from build123d import *

# Parameters (mm, degrees)
F1_DEPTH = 10
F3_DEPTH = 9
F4_R     = 2.5
F5_DEPTH = 9


with BuildPart() as f1:
    # F0 (on Right) → F1 (new body)
    with BuildSketch(Plane.YZ):
        Polygon((2.31229, 22.044512), (-24.890254, 22.044512), (-24.890254, 13.044512), (-0.099253, 13.044512), (23.129309, -0.366504), (27.629309, 7.427725), align=None)
    extrude(amount=F1_DEPTH)

    # F2 (on face) → F3 (join)
    with BuildSketch(Plane(origin=(0, 0, 13.044512), x_dir=(1, 0, 0), z_dir=(0, 0, -1))):
        with BuildLine():
            Line((0, 24.890254), (10, 24.890254))
            ThreePointArc((10, 24.890254), (5, 29.890254), (0, 24.890254))
        make_face()
    extrude(amount=-F3_DEPTH)

    # F4 (on face) → F5 (cut)
    with BuildSketch(Plane(origin=(0, 0, 13.044512), x_dir=(1, 0, 0), z_dir=(0, 0, -1))):
        with Locations((5, 24.890254)):
            Circle(F4_R)
    extrude(amount=-F5_DEPTH, mode=Mode.SUBTRACT)


solid = f1.part
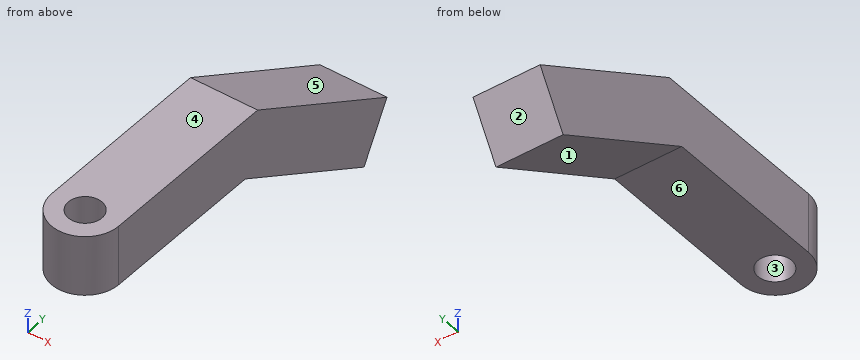
Part model, mm, in its own coordinate system. Face numbers are marked on the shaded views. A direction names the side the tool comes from. Give positions to 0.01 mm unless a question says otherwise; leave off trailing zeros. Order: outer loops, then holes, each group sorted by start corner. A loop starts at its lowest first (then second) coordinate and runs counter-clockwise, first axis right, second up. Notation, with made-up numbers: (-20.75, 50) - (-4.75, 50) arc R16 ccw to (-4.75, 67) - close; hole circle Ø6 at (7, 14). An arc over 180 degrees is marked (long way). Use a Markdown table: item, result.
1) Saw through at D-D on x = 1. List the corners of the cut face in (y, z), plus the area to 3 significant figures.
Checked values:
| item | result |
|---|---|
| outline | (-27.89, 13.04) - (-0.1, 13.04) - (23.13, -0.37) - (27.63, 7.43) - (2.31, 22.04) - (-27.89, 22.04) - close |
| area | 513 mm² |
2) 3-axis set-ups, long thin cutter, end or side, ignore diameter. For the marked faces 5 and 6: which of +Z, -Z, +X, -X, +Y, -Y reach the whole face in a straight line?
Checked values:
| item | result |
|---|---|
| face 5 | +Z, +X, -X, +Y |
| face 6 | -Z, +X, -X, -Y |
3) Saw through at A-A on x = 5. List the corners of the cut face in (y, z).
Checked values:
| item | result |
|---|---|
| outline | (-29.89, 13.04) - (-27.39, 13.04) - (-27.39, 22.04) - (-29.89, 22.04) - close; (-22.39, 13.04) - (-0.1, 13.04) - (23.13, -0.37) - (27.63, 7.43) - (2.31, 22.04) - (-22.39, 22.04) - close |
4) Two-plate mould, pull along Y, no slides. Class the marked faces 1, 2, 3 and 4: +Y half, -Y half, draft (parallel to the pull), parting line (faces both ways), or undercut.
Checked values:
| item | result |
|---|---|
| face 1 | -Y half |
| face 2 | +Y half |
| face 3 | undercut |
| face 4 | draft |
5) Saw through at C-C on y = -18.5. List the corners of the cut face in (x, z).
Checked values:
| item | result |
|---|---|
| outline | (0, 13.04) - (10, 13.04) - (10, 22.04) - (0, 22.04) - close |
6) Probe L1, parallel to Z at x = 3.25, y = -21.5; L2, parallel to Y at x = 5, z = 18; L3, parallel to Y at x = 5, z = 15.75. List the from-to ranges inside material, lowest first. Write a range as from..to.
Checked values:
| item | result |
|---|---|
| L1 | 13.04..22.04 |
| L2 | -29.89..-27.39, -22.39..9.32 |
| L3 | -29.89..-27.39, -22.39..13.21 |
7) Saw through at B-B on z = 15.25. List the corners of the cut face in (x, y), plus the area to 3 significant figures.
Checked values:
| item | result |
|---|---|
| outline | (0, -24.89) arc R5 ccw to (10, -24.89) - (10, 14.08) - (0, 14.08) - close; hole circle Ø5 at (5, -24.89) |
| area | 409 mm² |
8) Flat gauge pins, fed straight in: P1, Ø12, axis at y = -13.5, z = 19, coming from the -X side; P2, Ø1, axis at x = 3.5, y = -5.5, coming from the -Z side; P3, Ø8, axis at y = -6, z = 8, coming from the +X side; P4, Ø2, axis at x = 7.5, z = 17.5, coming from the -Y side. Where does each tip first touch, or does it go through?
Checked values:
| item | result |
|---|---|
| P1 | x = 0 |
| P2 | z = 13.04 |
| P3 | through |
| P4 | y = -29.66 |
